from build123d import *

# Parameters (mm, degrees)
SKETCH_1_R               = 2.75
EXTRUDE_1_DEPTH          = 2
SKETCH_2_R               = 1.5
EXTRUDE_2_DEPTH          = 6
CHAMFER_1_SIZE           = 0.2805
SKETCH_3_W               = 1.2
SKETCH_3_H               = 1.2
CUT_EXTRUDE_1_DEPTH      = 38
CUT_EXTRUDE_1_DEPTH_BACK = 38


with BuildPart() as part:
    # Sketch 1 → Extrude 1 (new body)
    with BuildSketch(Plane.XY):
        Circle(SKETCH_1_R)
    extrude(amount=EXTRUDE_1_DEPTH)

    # Sketch 2 → Extrude 2 (add)
    with BuildSketch(Plane(origin=(0, 0, 0), x_dir=(-1, 0, 0), z_dir=(0, 0, -1))):
        Circle(SKETCH_2_R)
    extrude(amount=EXTRUDE_2_DEPTH)

    # Chamfer 1
    chamfer_1_edges = [part.edges().sort_by_distance(p)[0] for p in [
        (1.5, 0, -6),
    ]]
    chamfer(chamfer_1_edges, length=CHAMFER_1_SIZE)

    # Sketch 3 → Cut-Extrude 1 (cut, two sides)
    with BuildSketch(Plane(origin=(0, 0, 0), x_dir=(1, 0, 0), z_dir=(0, 1, 0))) as cut_extrude_1_sk:
        with Locations((0, -2)):
            Rectangle(SKETCH_3_W, SKETCH_3_H)
    extrude(amount=CUT_EXTRUDE_1_DEPTH, mode=Mode.SUBTRACT)
    extrude(cut_extrude_1_sk.sketch, amount=-CUT_EXTRUDE_1_DEPTH_BACK, mode=Mode.SUBTRACT)


solid = part.part
Here's how the part is built. I have some questions about the finished solid (model axes, mm). A direction names the side the tool comes from. Give positions to 0.01 mm unless a question says otherwise; leave off trailing zeros. Order: outer loops, then holes, each group sorted by start corner. A loop starts at its lowest first (then second) coordinate and runs counter-clockwise, first axis right, second up. Notation, with made-up numbers: (-4, 43) -> (25, 43) arc R17 ccw to (25, 51) -> close; hole circle Ø8 at (-17, -14). An arc over 180 degrees is marked (long way). Use a Markdown table: item, result. Add a question column.
Item 1: I need wall thicknesses on line 1 (Z direction, x = 0.3, y = -1.8); line 2 (Z direction, x = 1.7, y = -2.05); line 3 (X direction, y = -0.6, z = 0.5). Which ranges of each line are inside material? Lowest first, please.
Item 2: Will these pins go through, and if not, where does the flat tip stop? pin 1 (0.6 mm diameter, centred on x = -0.5, y = 1, fed in from +Z); pin 2 (0.5 mm diameter, centred on y = 1, z = 1.5, fed in from -X); pin 3 (1 mm diameter, centred on y = -2, z = 0.5, fed in from +X); pin 4 (1 mm diameter, centred on x = -1.5, z = -3, fed in from -Y).
Item 3: Imagine slicing it at B-B on x = 0. Please give me the cut outline in (y, z), plus the area to 3 significant figures.
Item 4: Imagine slicing it at C-C on y = 0. Please give me the cut outline in (x, z).
Item 5: If we mould it in two halves opening along X, with no side actions, what happens to faces 3 (the face through (0, 0, 1.4)), 4 (the face through (2.62, 0.83, 0.99)), 5 (the face through (0, 0, -6))? For each: pulls with the +X half, pulls with the -X half, needs draft (parallel to the pull), parting line crosses it, or undercut.
Item 6: Imagine slicing it at D-D on z = 1. Please give me the cut outline in (x, y).
Item 7: For faces 1 (the face through (-1, 0, 2)), 2 (the face through (1.2, -1.2, 0)), which set-ups out of +Z, -Z, +X, -X, +Y, -Y let a thin tool reach every point of the face, with its end or its side?
Item 8: Imagine slicing it at A-A on y = 2.2. Please give me the cut outline in (x, z), plus the area to 3 significant figures.
Data:
| question | item | result |
|---|---|---|
| 1 | line 1 | z = 0 to 1.4 |
| 1 | line 2 | z = 0 to 2 |
| 1 | line 3 | x = -2.68 to 2.68 |
| 2 | pin 1 | stops at z = 2 |
| 2 | pin 2 | stops at x = -2.65 |
| 2 | pin 3 | stops at x = 2.3 |
| 2 | pin 4 | stops at y = -1.12 |
| 3 | outline | (-2.75, 0) -> (-1.5, 0) -> (-1.5, -5.72) -> (-1.22, -6) -> (1.22, -6) -> (1.5, -5.72) -> (1.5, 0) -> (2.75, 0) -> (2.75, 1.4) -> (-2.75, 1.4) -> close |
| 3 | area | 25.6 mm² |
| 4 | outline | (-2.75, 0) -> (-1.5, 0) -> (-1.5, -5.72) -> (-1.22, -6) -> (1.22, -6) -> (1.5, -5.72) -> (1.5, 0) -> (2.75, 0) -> (2.75, 2) -> (0.6, 2) -> (0.6, 1.4) -> (-0.6, 1.4) -> (-0.6, 2) -> (-2.75, 2) -> close |
| 5 | face 3 | undercut |
| 5 | face 4 | parting line crosses it |
| 5 | face 5 | needs draft |
| 6 | outline | circle Ø5.5 at (0, 0) |
| 7 | face 1 | +Z, +X, -X, +Y, -Y |
| 7 | face 2 | -Z |
| 8 | outline | (-1.65, 0) -> (1.65, 0) -> (1.65, 2) -> (0.6, 2) -> (0.6, 1.4) -> (-0.6, 1.4) -> (-0.6, 2) -> (-1.65, 2) -> close |
| 8 | area | 5.88 mm² |
